```python
from build123d import *

# Parameters (mm, degrees)
SKETCH4_R           = 10
BOSS_EXTRUDE2_DEPTH = 6


with BuildPart() as part:
    # Sketch1 → Revolve1 (revolve)
    with BuildSketch(Plane.XY, mode=Mode.PRIVATE) as revolve1_sk:
        with BuildLine():
            Line((20.9, 0), (23.871591838, 0))
            Line((23.871591838, 0), (23.871591838, 4))
            Line((23.871591838, 4), (22.9, 4.236662843))
            Line((22.9, 4.236662843), (22.9, 36.5))
            ThreePointArc((22.9, 36.5), (21.874873734, 38.974873734), (19.4, 40))
            Line((19.4, 40), (0, 40))
            Line((0, 40), (0, 38))
            Line((0, 38), (18.9, 38))
            ThreePointArc((18.9, 38), (20.314213562, 37.414213562), (20.9, 36))
            Line((20.9, 36), (20.9, 13.908178136))
            Line((20.9, 13.908178136), (0, 13.908178136))
            Line((0, 13.908178136), (0, 11.908178136))
            Line((0, 11.908178136), (20.9, 11.908178136))
            Line((20.9, 11.908178136), (20.9, 0))
        make_face()
    revolve(revolve1_sk.sketch.rotate(Axis((0, -0.724089275, 0), (0, 1, 0)), 90), axis=Axis((0, -0.724089275, 0), (0, 1, 0)))

    # Sketch4 → Boss-Extrude2 (add)
    with BuildSketch(Plane.XY.offset(22.9)):
        with Locations((1.144629865, 24.5)):
            Circle(SKETCH4_R)
    extrude(amount=-BOSS_EXTRUDE2_DEPTH)


solid = part.part
```
Here's how the part is built. I have some questions about the finished solid (model axes, mm). A direction names the side the tool comes from. Give positions to 0.01 mm unless a question says otherwise; leave off trailing zeros. Write each loop counter-clockwise with the first axis right and the second up, starting at its lowest first coordinate (ties: lowest second). Pieces come first, ordered by that corner, then holes. Notation, with made-up numbers: (33.5, -36) -> (92.5, -36) arc R31 cw to (92.5, -12) -> close; hole circle Ø3 at (-35.75, -24.5). An arc over 180 degrees is marked (long way). Write each question's results on one line, items separated by ' | '.
Item 1: We'd pull the mould along Y, two halves only. Please class faces 4 (the face through (0, 11.908, 0)), 5 (the face through (1, 25, 16.9)), 6 (the face through (-6.278, 5.871, -19.935)): pulls with the +Y half, pulls with the -Y half, needs draft (parallel to the pull), parting line crosses it, or undercut.
Output:
face 4: pulls with the -Y half | face 5: undercut | face 6: needs draft
Item 2: For pin 1 Ø8 at (y, z) = (15.5, 2.5) entering from +X; pin 2 Ø5 at (y, z) = (14.5, -10) entering from +X; pin 3 Ø10 at (x, y) = (-1.5, 24) entering from +Z, each with a flat end and sliding along its axis, tell me the tip position at first contact or that it passes through.
Output:
pin 1: stops at x = 22.9 | pin 2: stops at x = 21.64 | pin 3: stops at z = 22.9
Item 3: Suppose I cut it at C-C on y = 18.5. Write out the boundary of the cut face in (x, z), plus the area to 3 significant figures.
Output:
outline: (-6.86, 21.85) arc R22.9 ccw (long way) to (9.14, 20.99) -> (9.14, 22.9) -> (-6.86, 22.9) -> close; hole (-6.86, 16.9) -> (-6.86, 19.74) arc R20.9 ccw (long way) to (9.14, 18.79) -> (9.14, 16.9) -> close | area: 338 mm^2
Item 4: On a 3-axis mill with a long thin cutter (end or side, diameter ignored), from which of +Z, -Z, +X, -X, +Y, -Y can I reach the whole of each face in a straight line? I mean faces 1 (the face through (-6.278, 24.799, -19.935)), 2 (the face through (1, 25, 22.9)), 3 (the face through (0, 40, 0)). Say none if no direction works.
Output:
face 1: none | face 2: +Z, +X, -X, +Y | face 3: +Z, -Z, +X, -X, +Y
Item 5: If I drill on L1, parallel to Z at x = 0.5, y = 21; L2, parallel to Y at x = -4, z = -8; L3, parallel to X at y = 18, z = 0, over which ranges is the centre line in solid material (lowest first)?
Output:
L1: z = -22.89 to -20.89, 16.9 to 22.9 | L2: y = 11.91 to 13.91, 38 to 40 | L3: x = -22.9 to -20.9, 20.9 to 22.9
Item 6: Suppose I cut it at A-A on z = 0. Write out the boundary of the cut face in (x, y), plus the area to 3 significant figures.
Output:
outline: (-23.87, 0) -> (-20.9, 0) -> (-20.9, 11.91) -> (20.9, 11.91) -> (20.9, 0) -> (23.87, 0) -> (23.87, 4) -> (22.9, 4.24) -> (22.9, 36.5) arc R3.5 ccw to (19.4, 40) -> (-19.4, 40) arc R3.5 ccw to (-22.9, 36.5) -> (-22.9, 4.24) -> (-23.87, 4) -> close; hole (-20.9, 13.91) -> (20.9, 13.91) -> (20.9, 36) arc R2 ccw to (18.9, 38) -> (-18.9, 38) arc R2 ccw to (-20.9, 36) -> close | area: 332 mm^2
Item 7: Suppose I cut it at B-B on y = 24.5. Write out the boundary of the cut face in (x, z), plus the area to 3 significant figures.
Output:
outline: (-8.86, 21.12) arc R22.9 ccw (long way) to (11.14, 20.01) -> (11.14, 22.9) -> (-8.86, 22.9) -> close; hole (-8.86, 16.9) -> (-8.86, 18.93) arc R20.9 ccw (long way) to (11.14, 17.68) -> (11.14, 16.9) -> close | area: 354 mm^2
Item 8: Suppose I cut it at D-D on y = 3. Write out the boundary of the cut face in (x, z), plus the area to 3 significant figures.
Output:
outline: circle Ø47.74 at (0, 0); hole circle Ø41.8 at (0, 0) | area: 418 mm^2
